```python
from build123d import *

# Parameters (mm, degrees)
EXTRUDE_THIN1_DEPTH     = 7.5
SKETCH2_R               = 1.5
BOSS_EXTRUDE1_DEPTH     = 4
SKETCH3_R               = 3
CUT_EXTRUDE1_DEPTH      = 1
CUT_EXTRUDE1_DEPTH_BACK = 51


with BuildPart() as part:
    # Sketch1 → Extrude-Thin1 (new body, symmetric)
    with BuildSketch(Plane.XY):
        Polygon((-20, -15), (-20, 15), (20, 15), (20, -15), (25, -15), (25, 20), (-25, 20), (-25, -15), align=None)
    extrude(amount=EXTRUDE_THIN1_DEPTH, both=True)

    # Sketch2 → Boss-Extrude1 (add)
    with BuildSketch(Plane(origin=(0, 20, 0), x_dir=(1, 0, 0), z_dir=(0, 1, 0))):
        Circle(SKETCH2_R)
    extrude(amount=BOSS_EXTRUDE1_DEPTH)

    # Sketch3 → Cut-Extrude1 (cut, two sides)
    with BuildSketch(Plane(origin=(25, 0, 0), x_dir=(0, 0, -1), z_dir=(1, 0, 0))) as cut_extrude1_sk:
        with Locations((0, -5)):
            Circle(SKETCH3_R)
    extrude(amount=CUT_EXTRUDE1_DEPTH, mode=Mode.SUBTRACT)
    extrude(cut_extrude1_sk.sketch, amount=-CUT_EXTRUDE1_DEPTH_BACK, mode=Mode.SUBTRACT)


solid = part.part
```
CAD build for the part. Positions are in the model's coordinates, mm. A direction names the side the tool comes from. Coordinates: 2 decimals unless noted, no trailing zeros. Write each loop counter-clockwise with the first axis right and the second up, starting at its lowest first coordinate (ties: lowest second). Pieces come first, ordered by that corner, then holes.
(1) Two-plate mould, pull along X, no slides. Class faces 1 (the face through (-20, 0, 0)), 2 (the face through (0, 24, 0)), 3 (the face through (-1.5, 21.97, -0.07)): +X half, -X half, draft (parallel to the pull), parting line (faces both ways), or undercut.
(2) Cut at B-B, the plane z = 0. List the corners of the cut face in (x, y).
(3) 3-axis set-ups, long thin cutter, end or side, ignore diameter. For faces 4 (the face through (22, -15, 0)), 5 (the face through (0, 15, 0)): which of +Z, -Z, +X, -X, +Y, -Y reach the whole face in a straight line?
(4) Cut at C-C, the plane y = -5. List the corners of the cut face in (x, z).
(5) Cut at A-A, the plane y = -12. List the corners of the cut face in (x, z), and give its area (3 significant figures).
(6) Drill centre lines: probe 1 along X at (y, z) = (-12, 2.25); probe 2 along Y at (x, z) = (22.65, 0); probe 3 along Y at (x, z) = (-8, -6). Where is each one in solid material? Low to high.
(7) Cut at D-D, the plane x = 0. List the corners of the cut face in (y, z).
(8) Flat gauge pins, fed straight in: pin 1 (4.5 mm diameter, centred on x = -2, z = -2, fed in from -Y); pin 2 (7.5 mm diameter, centred on x = -5.5, z = 1.5, fed in from +Y); pin 3 (5.5 mm diameter, centred on y = -5, z = 0, fed in from -X). Where does each tip first touch, or does it go through?
Geometry says:
1. face 1: undercut
1. face 2: draft
1. face 3: parting line
2. outline: (-25, -15) - (-20, -15) - (-20, -8) - (-25, -8) - close; (-25, -2) - (-20, -2) - (-20, 15) - (20, 15) - (20, -2) - (25, -2) - (25, 20) - (1.5, 20) - (1.5, 24) - (-1.5, 24) - (-1.5, 20) - (-25, 20) - close; (20, -15) - (25, -15) - (25, -8) - (20, -8) - close
3. face 4: +Z, -Z, +X, -X, -Y
3. face 5: +Z, -Z, -Y
4. outline: (-25, -7.5) - (-20, -7.5) - (-20, -3) - (-25, -3) - close; (-25, 3) - (-20, 3) - (-20, 7.5) - (-25, 7.5) - close; (20, -7.5) - (25, -7.5) - (25, -3) - (20, -3) - close; (20, 3) - (25, 3) - (25, 7.5) - (20, 7.5) - close
5. outline: (-25, -7.5) - (-20, -7.5) - (-20, 7.5) - (-25, 7.5) - close; (20, -7.5) - (25, -7.5) - (25, 7.5) - (20, 7.5) - close
5. area: 150 mm2
6. probe 1: x = -25 to -20, 20 to 25
6. probe 2: y = -15 to -8, -2 to 20
6. probe 3: y = 15 to 20
7. outline: (15, -7.5) - (20, -7.5) - (20, -1.5) - (24, -1.5) - (24, 1.5) - (20, 1.5) - (20, 7.5) - (15, 7.5) - close
8. pin 1: stops at y = 15
8. pin 2: stops at y = 20
8. pin 3: passes through
